from build123d import *

# Parameters (mm, degrees)
SKETCH1_R           = 11.125
BOSS_EXTRUDE1_DEPTH = 8
BOSS_EXTRUDE2_DEPTH = 35


with BuildPart() as part:
    # Sketch1 → Boss-Extrude1 (new body)
    with BuildSketch(Plane.XY):
        Polygon((17.320508076, 0), (8.660254038, 15), (-8.660254038, 15), (-17.320508076, 0), (-8.660254038, -15), (8.660254038, -15), align=None)
        Circle(SKETCH1_R, mode=Mode.SUBTRACT)
    extrude(amount=-BOSS_EXTRUDE1_DEPTH)

    # Sketch2 → Boss-Extrude2 (add)
    with BuildSketch(Plane(origin=(0, 0, -8), x_dir=(-1, 0, 0), z_dir=(0, 0, -1))):
        with BuildLine():
            Line((-17.320508076, 0), (-10, 0))
            ThreePointArc((-10, 0), (0, -10), (10, 0))
            Line((10, 0), (17.320508076, 0))
            Line((17.320508076, 0), (8.660254038, -15))
            Line((8.660254038, -15), (-8.660254038, -15))
            Line((-8.660254038, -15), (-17.320508076, 0))
        make_face()
    extrude(amount=BOSS_EXTRUDE2_DEPTH)


solid = part.part
Input: part model. Units: mm. Frame: model coordinates. A direction names the side the tool comes from. Coordinates: 2 decimals unless noted, no trailing zeros. Loops run counter-clockwise (first coordinate to the right, second up) from the corner with the lowest first, then second, coordinate; pieces in that order, holes last. Notation, with made-up numbers: (-29, 78.5) -> (28, 78.5) arc R29 ccw to (28, 99.5) -> close; hole circle Ø11 at (51, 6). An arc over 180 degrees is marked (long way). Write each question's results on one line, items separated by ' | '. Start each with the question number.
Q1. Ray query, line 1 (Y direction, x = 0, z = -5) (3 decimals); line 2 (X direction, y = 0, z = -1.75) (1 decimal); line 3 (X direction, y = -7.5, z = -40.5). Return the intervals inside material, ascending. Write a range as from..to.
Q2. Section D-D, the plane y = 11.75. Return the cut outline in (x, z).
Q3. Section B-B, the plane y = 2.75. Return the cut outline in (x, z), plus the area to 3 significant figures.
Q4. Section A-A, the plane x = 0. Return the cut outline in (y, z) (3 decimals), plus the area to 3 significant figures.
Q5. Reachability of faces 4 (the flat face through (14, 0, -25)), 5 (the flat face through (-2, -10, -8)), 6 (the flat face through (0, -11, -43)) from +Z, -Z, +X, -X, +Y, -Y: full face, straight path, thin tool, end or side. Return the list, or none.
Q6. Pin query (flat end, axial travel): pin 1 (4 mm diameter, centred on x = -9.5, y = 2.5, fed in from +Z); pin 2 (2 mm diameter, centred on y = -3, z = -37, fed in from -X); pin 3 (6 mm diameter, centred on x = 14, z = -26, fed in from +Y); pin 4 (4 mm diameter, centred on x = -6.5, y = 0, fed in from +Z) (3 decimals). Return the tip coordinate at first contact, or that it passes through.
Q7. Pull-direction query (X, two-part tool) for faces 1 (the cylindrical face through (-8.2, 7.52, -3.94)), 2 (the flat face through (11.3, 0.2, 0)), 3 (the flat face through (-13.05, -7.4, -21.2)); classes: released by +X, released by -X, zero draft, split by the parting line, or undercut.
Q8. Section C-C, the plane z = -10. Return the cut outline in (x, y), plus the area to 3 significant figures.
Found:
1) line 1: -15..-11.125, 11.125..15 | line 2: -17.3..-11.1, 11.1..17.3 | line 3: -12.99..-6.61, 6.61..12.99
2) outline: (-10.54, -8) -> (10.54, -8) -> (10.54, 0) -> (-10.54, 0) -> close
3) outline: (-15.73, -8) -> (-10.78, -8) -> (-10.78, 0) -> (-15.73, 0) -> close; (10.78, -8) -> (15.73, -8) -> (15.73, 0) -> (10.78, 0) -> close | area: 79.2 mm2
4) outline: (-15, -43) -> (-10, -43) -> (-10, -8) -> (-11.125, -8) -> (-11.125, 0) -> (-15, 0) -> close; (11.125, -8) -> (15, -8) -> (15, 0) -> (11.125, 0) -> close | area: 237 mm2
5) face 4: -Z, +X, -X, +Y | face 5: +Z | face 6: -Z, +X, -X, +Y, -Y
6) pin 1: z = 0 | pin 2: x = -16.17 | pin 3: y = 0 | pin 4: through
7) face 1: undercut | face 2: zero draft | face 3: released by -X
8) outline: (-17.32, 0) -> (-8.66, -15) -> (8.66, -15) -> (17.32, 0) -> (10, 0) arc R10 cw to (-10, 0) -> close | area: 233 mm2
